Input: part model. Units: mm. Frame: model coordinates. A direction names the side the tool comes from. Round coordinates to 2 decimals unless told otherwise and drop trailing zeros. Loops run counter-clockwise (first coordinate to the right, second up) from the corner with the lowest first, then second, coordinate; pieces in that order, holes last. Notation, with made-up numbers: (54, 66) - (105, 66) arc R13 cw to (105, 71) - close; hole circle Ø1 at (-11.5, 69). An arc over 180 degrees is marked (long way). Write each question's results on one line, items separated by ' | '.
from build123d import *

# Parameters (mm, degrees)
SKETCH1_R           = 1.5875
BOSS_EXTRUDE1_DEPTH = 1.5875


with BuildPart() as part:
    # Sketch1 → Boss-Extrude1 (new body)
    with BuildSketch(Plane.XY):
        with BuildLine():
            Line((-40.64, 20.32), (-40.64, 26.035))
            ThreePointArc((-40.64, 26.035), (-39.896051224, 27.831051224), (-38.1, 28.575))
            Line((-38.1, 28.575), (-27.94, 28.575))
            Line((-27.94, 28.575), (-27.94, 31.75))
            ThreePointArc((-27.94, 31.75), (-27.14625, 32.54375), (-26.3525, 31.75))
            Line((-26.3525, 31.75), (-26.3525, 28.575))
            Line((-26.3525, 28.575), (26.3525, 28.575))
            Line((26.3525, 28.575), (26.3525, 31.75))
            ThreePointArc((26.3525, 31.75), (27.14625, 32.54375), (27.94, 31.75))
            Line((27.94, 31.75), (27.94, 28.575))
            Line((27.94, 28.575), (38.1, 28.575))
            ThreePointArc((38.1, 28.575), (39.896051224, 27.831051224), (40.64, 26.035))
            Line((40.64, 26.035), (40.64, 20.32))
            Line((40.64, 20.32), (46.99, 20.32))
            Line((46.99, 20.32), (46.99, 27.305))
            ThreePointArc((46.99, 27.305), (44.758153673, 32.693153673), (39.37, 34.925))
            Line((39.37, 34.925), (-39.37, 34.925))
            ThreePointArc((-39.37, 34.925), (-44.758153673, 32.693153673), (-46.99, 27.305))
            Line((-46.99, 27.305), (-46.99, 20.32))
            Line((-46.99, 20.32), (-40.64, 20.32))
        make_face()
        with Locations((-43.815, 23.495)):
            Circle(SKETCH1_R, mode=Mode.SUBTRACT)
        with Locations((43.815, 23.495)):
            Circle(SKETCH1_R, mode=Mode.SUBTRACT)
    extrude(amount=BOSS_EXTRUDE1_DEPTH)


solid = part.part
1. Contact query for flat-ended pins moving along their axis: pin 1 (0.5 mm diameter, centred on y = 30, z = 1, fed in from +X); pin 2 (0.8 mm diameter, centred on x = 30.5, z = 1, fed in from -Y) (3 decimals); pin 3 (0.5 mm diameter, centred on y = 30.5, z = 1, fed in from +X); pin 4 (3 mm diameter, centred on x = -43.815, y = 23.495, fed in from -Z). Output: stop coordinate, or through.
Answer:
pin 1: x = 46.59 | pin 2: y = 28.575 | pin 3: x = 46.4 | pin 4: through
2. Section query A-A, the plane x = 37. Output: boundary loops of the cut face in (y, z) (1 decimal), plus the area to 3 significant figures.
Answer:
outline: (28.6, 0) - (34.9, 0) - (34.9, 1.6) - (28.6, 1.6) - close | area: 10.1 mm^2
3. Section query B-B, the plane z = 0.9. Count the separate pieces of the cut face and the enclosed holes in it, plus the area to 3 significant figures.
Answer:
separate pieces: 1 | enclosed holes: 2 | area: 652 mm^2
4. Section query C-C, the plane y = 33.5. Output: boundary loops of the cut face in (x, z).
Answer:
outline: (-43.81, 0) - (43.81, 0) - (43.81, 1.59) - (-43.81, 1.59) - close
5. Mould query, pull axis Y, two halves, no side actions, for faces 1 (the flat face through (27.94, 30, 1)), 2 (the cylindrical face through (-44.7, 32.75, 0.78)), 3 (the cylindrical face through (-39.916, 27.811, 0.783)), 4 (the cylindrical face through (44.668, 24.834, 0.783)). Classes: pulls with the +Y half, pulls with the -Y half, needs draft (parallel to the pull), parting line crosses it, or undercut.
Answer:
face 1: needs draft | face 2: pulls with the +Y half | face 3: pulls with the -Y half | face 4: undercut
6. Set-up query: faces 5 (the flat face through (1, 34.925, 1)), 6 (the flat face through (33, 28.575, 1)). Return all of +Z, -Z, +X, -X, +Y, -Y with unobstructed straight access to the full face (end or side cutting, diameter ignored); none if empty.
Answer:
face 5: +Z, -Z, +X, -X, +Y | face 6: +Z, -Z, -Y
7. Line query: line 1 (X direction, y = 23.5, z = 1.55); line 2 (X direction, y = 22.5, z = 0.15); line 3 (X direction, y = 21.5, z = 0.3). Output: solid intervals per line, ascending. Write a range as [from, to].
Answer:
line 1: [-46.99, -45.4], [-42.23, -40.64], [40.64, 42.23], [45.4, 46.99] | line 2: [-46.99, -45.05], [-42.58, -40.64], [40.64, 42.58], [45.05, 46.99] | line 3: [-46.99, -40.64], [40.64, 46.99]
